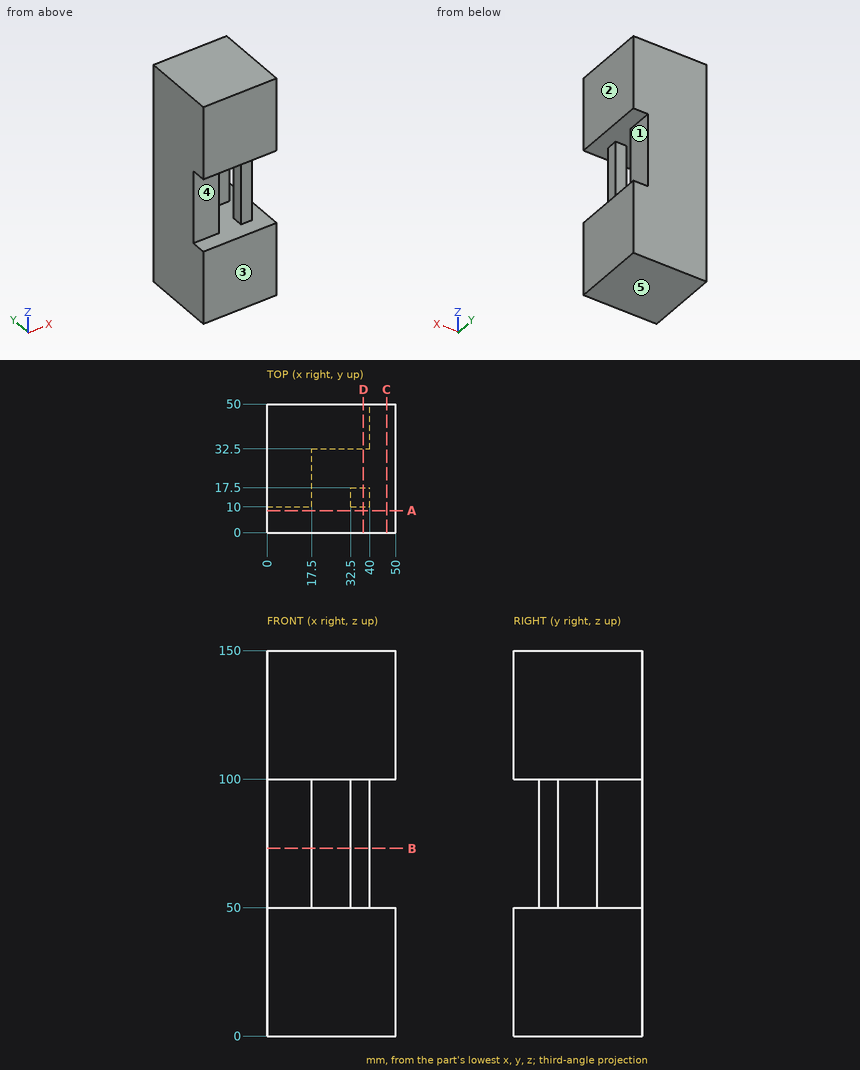
Source: three-view drawing plus pictorial views. Frame: mm from the lowest corner of the part. A direction names the side the tool comes from. Give positions to 0.01 mm unless a question says otherwise; leave off trailing zeros. Loops run counter-clockwise (first coordinate to the right, second up) from the corner with the lowest first, then second, coordinate; pieces in that order, holes last. Notation, with made-up numbers: M 9.5,29 L 67.5,29 A24 cw 67.5,56 Z; hole C 30,-9.5 d9. An arc over 180 degrees is marked long. Put each result on its own line as item: value.
Q1. Section A-A (y = 8.5). Return the cut outline in (x, z), and give its area (3 significant figures).
Response values:
outline: M 0,0 L 50,0 L 50,50 L 0,50 Z; M 0,100 L 50,100 L 50,150 L 0,150 Z
area: 5,000 mm²
Q2. Pin query (flat end, axial travel): P1, Ø4, axis at x = 35.5, z = 73.5, coming from the -Y side; P2, Ø1, axis at x = 21.5, z = 72.5, coming from the -Y side; P3, Ø8, axis at y = 12.5, z = 78, coming from the +X side. Return the tip coordinate at first contact, or that it passes through.
Response values:
P1: stops at y = 10
P2: stops at y = 32.5
P3: stops at x = 40
Q3. Reachability of the marked faces 1 and 2 from +Z, -Z, +X, -X, +Y, -Y: full face, straight path, thin tool, end or side. Return the list, or none.
Response values:
face 1: +X, +Y, -Y
face 2: +Z, -Z, +X, +Y, -Y
Q4. Line query: probe 1 along Z at (x, y) = (25, 5.5); probe 2 along X at (y, z) = (11, 60); probe 3 along Y at (x, z) = (38, 82). Output: solid intervals per line, ascending. Write a range as [from, to].
Response values:
probe 1: z = [0, 50], [100, 150]
probe 2: x = [0, 17.5], [32.5, 40]
probe 3: y = [10, 17.5], [32.5, 50]
Q5. Mould query, pull axis Z, two halves, no side actions, for the marked faces 3, 4 and 5. Classes: released by +Z, released by -Z, zero draft, split by the parting line, or undercut.
Response values:
face 3: zero draft
face 4: undercut
face 5: released by -Z
Q6. Section B-B (z = 73). Return the cut outline in (x, y), and give its area (3 significant figures).
Response values:
outline: M 0,10 L 17.5,10 L 17.5,32.5 L 40,32.5 L 40,50 L 0,50 Z; M 32.5,10 L 40,10 L 40,17.5 L 32.5,17.5 Z
area: 1,150 mm²
Q7. Section D-D (x = 37.5). Return the cut outline in (y, z), and give its area (3 significant figures).
Response values:
outline: M 0,0 L 50,0 L 50,150 L 0,150 L 0,100 L 10,100 L 10,50 L 0,50 Z; hole M 17.5,50 L 32.5,50 L 32.5,100 L 17.5,100 Z
area: 6,250 mm²
